Can you work these out from the model? Positions are in its coordinate system, mm. A direction names the side the tool comes from. Give positions to 0.01 mm unless a question says otherwise; leave off trailing zeros. Order: outer loops, then holes, each group sorted by start corner. A loop starts at its lowest first (then second) coordinate and runs counter-clockwise, first axis right, second up. Notation, with made-up numbers: M 45,-18.5 L 61,-18.5 A8 ccw 61,-11.5 Z; hole C 34.5,-22 d8. An arc over 180 degrees is marked long. Use one line per item in the form item = value. Start each with the question number.
1. I need wall thicknesses on L1, parallel to X at y = 9.25, z = 2.5; L2, parallel to Z at x = 4.5, y = 13.75; L3, parallel to Y at x = 2, z = 18.5. Which ranges of each line are inside material? Lowest first, please.
2. I want a section at C-C, the plane y = 7. List the corners of the cut face in (x, z) for me.
3. I want a section at A-A, the plane y = 9.9. List the corners of the cut face in (x, z) for me (3 decimals), and give its area (3 significant figures).
4. Will these pins go through, and if not, where does the flat tip stop? P1, Ø2, axis at y = 11, z = -1.5, coming from the -X side; P2, Ø1.6, axis at x = -13.64, y = 9.9, coming from the +Z side; P3, Ø4, axis at x = -13.5, z = -4.5, coming from the +Y side; P4, Ø4.5, axis at x = -15.5, y = 11.5, coming from the +Z side.
5. I want a section at B-B, the plane x = -5.31. List the corners of the cut face in (y, z) for me (3 decimals).
6. I want a section at D-D, the plane x = -16. List the corners of the cut face in (y, z) for me.
7. For faces 1 (the face through (-20, 3, -4)), 2 (the face through (-6, 6, -16)), 3 (the face through (-13.107, 10.743, 2.638)), 4 (the face through (11.26, 8, 3)), 5 (the face through (16, 10, 0.762)), which set-ups out of +Z, -Z, +X, -X, +Y, -Y let a thin tool reach every point of the face, with its end or its side?
8. We'd pull the mould along X, two halves only. Please class faces 6 (the face through (9.38, 8, -18)), 7 (the face through (-17.5, 2, -8.2)), 8 (the face through (-19.14, 14.9, 2.59)), 9 (the face through (12.66, 9.94, 2.64)): +X half, -X half, draft (parallel to the pull), parting line (faces both ways), or undercut.
```python
from build123d import *

# Parameters (mm, degrees)
SKETCH1_W           = 40
SKETCH1_H           = 40
BOSS_EXTRUDE1_DEPTH = 4
SKETCH2_W           = 8.739547094
SKETCH2_H           = 3.7
BOSS_EXTRUDE2_DEPTH = 11.8
BOSS_EXTRUDE3_DEPTH = 11.8
SKETCH4_R           = 3.745
CUT_EXTRUDE1_DEPTH  = 5
SKETCH5_R           = 1
CUT_EXTRUDE2_DEPTH  = 3.7
SKETCH6_R           = 1.5
CUT_EXTRUDE3_DEPTH  = 5
FILLET1_R           = 3
FILLET2_R           = 3


with BuildPart() as part:
    # Sketch1 → Boss-Extrude1 (new body)
    with BuildSketch(Plane(origin=(0, 0, 0), x_dir=(1, 0, 0), z_dir=(0, 1, 0))):
        Rectangle(SKETCH1_W, SKETCH1_H)
    extrude(amount=BOSS_EXTRUDE1_DEPTH)

    # Sketch2 → Boss-Extrude2 (add)
    with BuildSketch(Plane(origin=(0, 4, 0), x_dir=(1, 0, 0), z_dir=(0, 1, 0))):
        Polygon((-20, -0.761716699), (-11.276069587, -0.761716699), (-11.244836225, -4.461716699), (-20, -4.461716699), align=None)
        with Locations((15.630226453, -2.611716699)):
            Rectangle(SKETCH2_W, SKETCH2_H)
    extrude(amount=BOSS_EXTRUDE2_DEPTH)

    # Sketch3 → Boss-Extrude3 (add)
    with BuildSketch(Plane(origin=(0, 4, 0), x_dir=(1, 0, 0), z_dir=(0, 1, 0))):
        Polygon((9.38, 16), (-5.31, 16), (-20, 16), (-20, 20), (-5.31, 20), (9.38, 20), align=None)
    extrude(amount=BOSS_EXTRUDE3_DEPTH)

    # Sketch4 → Cut-Extrude1 (cut, through all)
    with BuildSketch(Plane.XY.offset(-16)):
        with Locations((-5.31, 9.9)):
            Circle(SKETCH4_R)
    extrude(amount=-CUT_EXTRUDE1_DEPTH, mode=Mode.SUBTRACT)

    # Sketch5 → Cut-Extrude2 (cut)
    with BuildSketch(Plane.XY.offset(4.461716699)):
        with Locations((-13.644836225, 9.9)):
            Circle(SKETCH5_R)
        with Locations((13.660452906, 9.9)):
            Circle(SKETCH5_R)
    extrude(amount=-CUT_EXTRUDE2_DEPTH, mode=Mode.SUBTRACT)

    # Sketch6 → Cut-Extrude3 (cut, through all)
    with BuildSketch(Plane(origin=(0, 4, 0), x_dir=(1, 0, 0), z_dir=(0, 1, 0))):
        with Locations((15.757359313, 15.757359313)):
            Circle(SKETCH6_R)
        with Locations((15.757359313, -15.757359313)):
            Circle(SKETCH6_R)
        with Locations((-16, 8.145789662)):
            Circle(SKETCH6_R)
    extrude(amount=-CUT_EXTRUDE3_DEPTH, mode=Mode.SUBTRACT)

    # Fillet1
    fillet1_edges = [part.edges().sort_by_distance(p)[0] for p in [
        (-11.260452906, 15.8, 2.611716699),
        (-20, 15.8, 2.611716699),
        (20, 15.8, 2.611716699),
        (11.260452906, 15.8, 2.611716699),
        (9.38, 15.8, -18),
        (-20, 15.8, -18),
    ]]
    fillet(fillet1_edges, radius=FILLET1_R)

    # Fillet2
    fillet2_edges = [part.edges().sort_by_distance(p)[0] for p in [
        (20, 2, 20),
        (20, 2, -20),
    ]]
    fillet(fillet2_edges, radius=FILLET2_R)


solid = part.part
```
Check result:
q1.L1 = -20 to -14.4, -12.88 to -11.26, 11.26 to 12.9, 14.42 to 20
q1.L2 = -20 to -16
q1.L3 = 0 to 4
q2.outline = M -20,-20 L -7.68,-20 L -7.68,-16 L -20,-16 Z; M -20,0.76 L -11.28,0.76 L -11.24,4.46 L -20,4.46 Z; M -2.94,-20 L 9.38,-20 L 9.38,-16 L -2.94,-16 Z; M 11.26,0.76 L 20,0.76 L 20,4.46 L 11.26,4.46 Z
q3.outline = M -20,-20 L -9.055,-20 L -9.055,-16 L -20,-16 Z; M -20,0.762 L -14.645,0.762 L -14.645,4.462 L -20,4.462 Z; M -12.645,0.762 L -11.276,0.762 L -11.245,4.462 L -12.645,4.462 Z; M -1.565,-20 L 9.38,-20 L 9.38,-16 L -1.565,-16 Z; M 11.26,0.762 L 12.66,0.762 L 12.66,4.462 L 11.26,4.462 Z; M 14.66,0.762 L 20,0.762 L 20,4.462 L 14.66,4.462 Z
q3.area = 137 mm2
q4.P1 = through
q4.P2 = -16
q4.P3 = 4
q4.P4 = 4.46
q5.outline = M 0,-20 L 6.155,-20 L 6.155,-16 L 4,-16 L 4,20 L 0,20 Z; M 13.645,-20 L 15.8,-20 L 15.8,-16 L 13.645,-16 Z
q6.outline = M 0,-20 L 15.8,-20 L 15.8,-16 L 4,-16 L 4,-9.65 L 0,-9.65 Z; M 0,-6.65 L 4,-6.65 L 4,0.76 L 15.8,0.76 L 15.8,4.46 L 4,4.46 L 4,20 L 0,20 Z
q7.face_1 = +Z, -Z, -X, +Y, -Y
q7.face_2 = +X, -X, +Y
q7.face_3 = +Z
q7.face_4 = +Z, -Z, +Y
q7.face_5 = -Z, +X, -X, +Y
q8.face_6 = +X half
q8.face_7 = undercut
q8.face_8 = -X half
q8.face_9 = undercut
